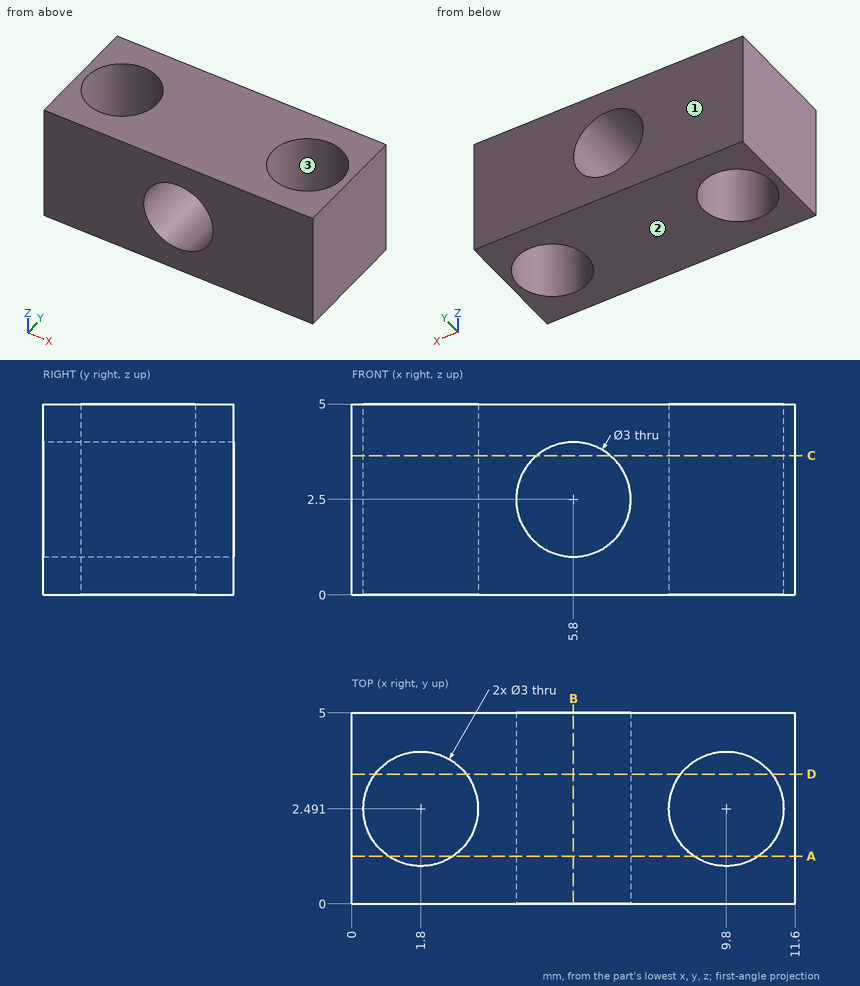
Verification items for this drawing (mm, ordinates from the low corner). Coordinates: 2 decimals unless noted, no trailing zeros. Write each loop counter-clockwise with the first axis right and the second up, starting at its lowest first coordinate (ties: lowest second). Pieces come first, ordered by that corner, then holes. Notation, with made-up numbers: M -10,-32.5 L 30,-32.5 A25 cw 30,-8.5 Z; hole C -3.75,79 d7. An arc over 180 degrees is marked long. Answer as a JSON object with one key per item and string values. Group by question number.
(1) Cross-section at A-A, the plane y = 1.25. Record the cut outline in (x, z).
(2) Material ranges on line 1 (Y direction, x = 1.75, z = 3.65); line 2 (X direction, y = 1.65, z = 2.5); line 3 (X direction, y = 1.9, z = 2.5), recorded low to high.
(3) Cross-section at C-C, the plane z = 3.65. Record the cut outline in (x, y).
(4) Cross-section at D-D, the plane y = 3.4. Record the cut outline in (x, z).
(5) Release check for a two-part mould opening along Y. For the marked faces 1, 2 and 3 record: +Y half, -Y half, draft (parallel to the pull), parting line (faces both ways), or undercut.
(6) Cross-section at B-B, the plane x = 5.8. Record the cut outline in (y, z).
Reply:
{
 "1": {"outline": "M 0,0 L 0.96,0 L 0.96,5 L 0,5 Z; M 2.64,0 L 8.96,0 L 8.96,5 L 2.64,5 Z; M 10.64,0 L 11.6,0 L 11.6,5 L 10.64,5 Z; hole C 5.8,2.5 d3"},
 "2": {"line 1": "0 to 0.99, 3.99 to 5", "line 2": "0 to 0.56, 3.04 to 4.3, 7.3 to 8.56, 11.04 to 11.6", "line 3": "0 to 0.42, 3.18 to 4.3, 7.3 to 8.42, 11.18 to 11.6"},
 "3": {"outline": "M 0,0 L 4.84,0 L 4.84,5 L 0,5 Z; M 6.76,0 L 11.6,0 L 11.6,5 L 6.76,5 Z; hole C 1.8,2.49 d3; hole C 9.8,2.49 d3"},
 "4": {"outline": "M 0,0 L 0.61,0 L 0.61,5 L 0,5 Z; M 2.99,0 L 8.61,0 L 8.61,5 L 2.99,5 Z; M 10.99,0 L 11.6,0 L 11.6,5 L 10.99,5 Z; hole C 5.8,2.5 d3"},
 "5": {"face 1": "+Y half", "face 2": "draft", "face 3": "undercut"},
 "6": {"outline": "M 0,0 L 5,0 L 5,1 L 0,1 Z; M 0,4 L 5,4 L 5,5 L 0,5 Z"}
}
